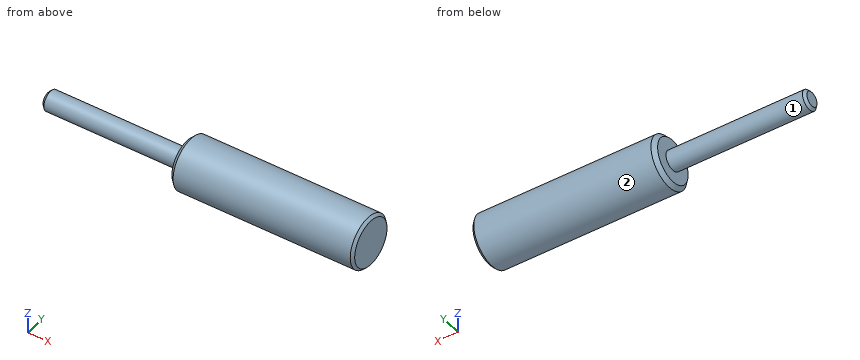
```python
from build123d import *

# Parameters (mm, degrees)
SKETCH_1_R      = 9.8
EXTRUDE_1_DEPTH = 70
SKETCH_2_R      = 3.75
EXTRUDE_2_DEPTH = 53
CHAMFER_1_SIZE  = 1.5
CHAMFER_2_SIZE  = 1
CHAMFER_3_SIZE  = 1


with BuildPart() as part:
    # 草图1 → 凸台-拉伸1 (new body)
    with BuildSketch(Plane(origin=(0, 0, 0), x_dir=(0, 0, -1), z_dir=(1, 0, 0))):
        Circle(SKETCH_1_R)
    extrude(amount=EXTRUDE_1_DEPTH)

    # 草图2 → 凸台-拉伸2 (add)
    with BuildSketch(Plane.ZY):
        Circle(SKETCH_2_R)
    extrude(amount=EXTRUDE_2_DEPTH)

    # 倒角1
    chamfer_1_edges = [part.edges().sort_by_distance(p)[0] for p in [
        (0, 0, 9.8),
    ]]
    chamfer(chamfer_1_edges, length=CHAMFER_1_SIZE)

    # 倒角2
    chamfer_2_edges = [part.edges().sort_by_distance(p)[0] for p in [
        (-53, 0, -3.75),
    ]]
    chamfer(chamfer_2_edges, length=CHAMFER_2_SIZE)

    # 倒角3
    chamfer_3_edges = [part.edges().sort_by_distance(p)[0] for p in [
        (70, 0, 9.8),
    ]]
    chamfer(chamfer_3_edges, length=CHAMFER_3_SIZE)


solid = part.part
```
The listing builds one solid part. Answer for the finished solid, in the listing's coordinates (mm). Face numbers are marked on the shaded views. A direction names the side the tool comes from. Give positions to 0.01 mm unless a question says otherwise; leave off trailing zeros. Order: outer loops, then holes, each group sorted by start corner. A loop starts at its lowest first (then second) coordinate and runs counter-clockwise, first axis right, second up. Notation, with made-up numbers: (-5.5, 38) - (8.5, 38) arc R6 cw to (8.5, 43) - close; hole circle Ø9 at (-9, 45). An arc over 180 degrees is marked (long way). Answer in a Markdown table with one row per item. Add a question column.
Q1. Find the intervals of material crossed by line 1 along X through (y, z) = (5, 3); line 2 along Y through (x, z) = (62, 0); line 3 along Y through (x, z) = (-7, 0), in increasing order. Write a range as [from, to].
Q2. The part is cut by section A-A (y = 0). Determine the outline of the cut face in (x, z), then the cut area to 3 significant figures.
Q3. Which of the six approach directions +Z, -Z, +X, -X, +Y, -Y give full straight-line access (tool end or side, diameter ignored) to the marked faces 1 and 2?
Q4. The part is cut by section D-D (x = 32.5). Determine the outline of the cut face in (y, z).
Q5. The part is cut by section C-C (x = -15). Determine the outline of the cut face in (y, z), then the cut area to 3 significant figures.
Q6. Given P1, Ø8, axis at x = -5.5, y = -7, coming from the -Z side; P2, Ø6, axis at x = -24, z = 1, coming from the -Y side; P3, Ø8, axis at x = -11.5, y = 0, coming from the -Z side, each flat-ended and moving along its own axis, determine where each tip first touches the part or whether it passes through.
Determined:
| question | item | result |
|---|---|---|
| 1 | line 1 | x = [0, 70] |
| 1 | line 2 | y = [-9.8, 9.8] |
| 1 | line 3 | y = [-3.75, 3.75] |
| 2 | outline | (-53, -2.75) - (-52, -3.75) - (0, -3.75) - (0, -8.3) - (1.5, -9.8) - (69, -9.8) - (70, -8.8) - (70, 8.8) - (69, 9.8) - (1.5, 9.8) - (0, 8.3) - (0, 3.75) - (-52, 3.75) - (-53, 2.75) - close |
| 2 | area | 1,770 mm² |
| 3 | face 1 | -X |
| 3 | face 2 | +X, -X |
| 4 | outline | circle Ø19.6 at (0, 0) |
| 5 | outline | circle Ø7.5 at (0, 0) |
| 5 | area | 44.2 mm² |
| 6 | P1 | stops at z = -2.25 |
| 6 | P2 | stops at y = -3.75 |
| 6 | P3 | stops at z = -3.75 |
